```python
from build123d import *

# Parameters (mm, degrees)
SKETCH_1_R               = 30
SKETCH_1_R_2             = 2.75
EXTRUDE_1_DEPTH          = 5
SKETCH_2_R               = 12
EXTRUDE_2_DEPTH          = 10
SKETCH_3_R               = 6
EXTRUDE_3_DEPTH          = 10
SKETCH_5_R               = 5
EXTRUDE_4_DEPTH          = 24.1
SKETCH_6_R               = 2
CUT_EXTRUDE_1_DEPTH      = 10
CUT_EXTRUDE_1_DEPTH_BACK = 10


with BuildPart() as part:
    # Sketch 1 → Extrude 1 (new body)
    with BuildSketch(Plane.XY):
        Circle(SKETCH_1_R)
        with Locations((0, 22.5)):
            Circle(SKETCH_1_R_2, mode=Mode.SUBTRACT)
        with Locations((19.485571585, 11.25)):
            Circle(SKETCH_1_R_2, mode=Mode.SUBTRACT)
        with Locations((19.485571585, -11.25)):
            Circle(SKETCH_1_R_2, mode=Mode.SUBTRACT)
        with Locations((0, -22.5)):
            Circle(SKETCH_1_R_2, mode=Mode.SUBTRACT)
        with Locations((-19.485571585, -11.25)):
            Circle(SKETCH_1_R_2, mode=Mode.SUBTRACT)
        with Locations((-19.485571585, 11.25)):
            Circle(SKETCH_1_R_2, mode=Mode.SUBTRACT)
    extrude(amount=EXTRUDE_1_DEPTH)

    # Sketch 2 → Extrude 2 (add)
    with BuildSketch(Plane.XY.offset(5)):
        Circle(SKETCH_2_R)
    extrude(amount=EXTRUDE_2_DEPTH)

    # Sketch 3 → Extrude 3 (add)
    with BuildSketch(Plane.XY.offset(15)):
        Circle(SKETCH_3_R)
    extrude(amount=EXTRUDE_3_DEPTH)

    # Sketch 5 → Extrude 4 (add)
    with BuildSketch(Plane.XY.offset(25)):
        Circle(SKETCH_5_R)
    extrude(amount=EXTRUDE_4_DEPTH)

    # Sketch 6 → Cut-Extrude 1 (cut, two sides)
    with BuildSketch(Plane(origin=(0, 0, 0), x_dir=(1, 0, 0), z_dir=(0, 1, 0))) as cut_extrude_1_sk:
        with Locations((0, -39.1)):
            Circle(SKETCH_6_R)
    extrude(amount=CUT_EXTRUDE_1_DEPTH, mode=Mode.SUBTRACT)
    extrude(cut_extrude_1_sk.sketch, amount=-CUT_EXTRUDE_1_DEPTH_BACK, mode=Mode.SUBTRACT)


solid = part.part
```
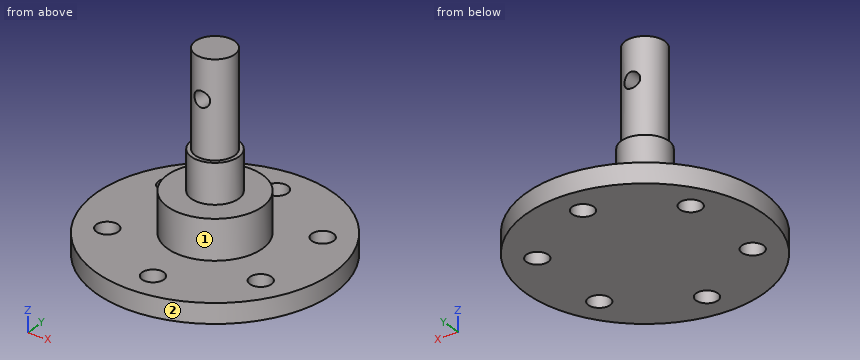
Design review of the part built by this model. Coordinates are the model's own, in mm. Face numbers are marked on the shaded views. A direction names the side the tool comes from. Give positions to 0.01 mm unless a question says otherwise; leave off trailing zeros. Order: outer loops, then holes, each group sorted by start corner. A loop starts at its lowest first (then second) coordinate and runs counter-clockwise, first axis right, second up. Notation, with made-up numbers: (72, -13.75) -> (102, -13.75) arc R31 cw to (102, 24.25) -> close; hole circle Ø2 at (87, 22). An arc over 180 degrees is marked (long way). Write each question's results on one line, items separated by ' | '. Start each with the question number.
Q1. Machinability: for the marked faces 1 and 2, which of the approach directions +Z, -Z, +X, -X, +Y, -Y give a long, thin tool a straight path to every point of the face, cutting with its end or side? Answer none if there is none.
Q2. Add section A-A on x = 0. Give the boundary of the cut face in (y, z), and give its area (3 significant figures).
Q3. Add section D-D on x = -18.5. Give the boundary of the cut face in (y, z).
Q4. Wall thickness on L1, parallel to Y at x = 0, z = 3.05; L2, parallel to X at y = -11, z = 3; L3, parallel to Z at x = 21, y = 16.5: over which ranges is each line inside the solid? List them lowest first. Write a range as from..to.
Q5. For pin 1 (3.5 mm diameter, centred on x = -19.49, y = 11.25, fed in from +Z); pin 2 (2 mm diameter, centred on x = 4, y = 10.5, fed in from +Z); pin 3 (12 mm diameter, centred on x = -5, z = 26.5, fed in from +Y); pin 4 (6 mm diameter, centred on x = -22.5, z = 7.5, fed in from -Y), all flat-tipped, find the tip position at first contact; note any pin that passes through.
Q6. Add section C-C on y = 0. Give the boundary of the cut face in (x, z).
Q7. Add section B-B on y = -13. Give the boundary of the cut face in (x, z).
Found:
1) face 1: +Z | face 2: +Z, -Z
2) outline: (-30, 0) -> (-25.25, 0) -> (-25.25, 5) -> (-30, 5) -> close; (-19.75, 0) -> (19.75, 0) -> (19.75, 5) -> (12, 5) -> (12, 15) -> (6, 15) -> (6, 25) -> (5, 25) -> (5, 37.1) -> (-5, 37.1) -> (-5, 25) -> (-6, 25) -> (-6, 15) -> (-12, 15) -> (-12, 5) -> (-19.75, 5) -> close; (-5, 41.1) -> (5, 41.1) -> (5, 49.1) -> (-5, 49.1) -> close; (25.25, 0) -> (30, 0) -> (30, 5) -> (25.25, 5) -> close | area: 806 mm2
3) outline: (-23.62, 0) -> (-13.82, 0) -> (-13.82, 5) -> (-23.62, 5) -> close; (-8.68, 0) -> (8.68, 0) -> (8.68, 5) -> (-8.68, 5) -> close; (13.82, 0) -> (23.62, 0) -> (23.62, 5) -> (13.82, 5) -> close
4) L1: y = -30..-25.25, -19.75..19.75, 25.25..30 | L2: x = -27.91..-22.22, -16.75..16.75, 22.22..27.91 | L3: z = 0..5
5) pin 1: passes through | pin 2: stops at z = 15 | pin 3: stops at y = 6 | pin 4: stops at y = -21.58
6) outline: (-30, 0) -> (30, 0) -> (30, 5) -> (12, 5) -> (12, 15) -> (6, 15) -> (6, 25) -> (5, 25) -> (5, 49.1) -> (-5, 49.1) -> (-5, 25) -> (-6, 25) -> (-6, 15) -> (-12, 15) -> (-12, 5) -> (-30, 5) -> close; hole circle Ø4 at (0, 39.1)
7) outline: (-27.04, 0) -> (-21.61, 0) -> (-21.61, 5) -> (-27.04, 5) -> close; (-17.36, 0) -> (17.36, 0) -> (17.36, 5) -> (-17.36, 5) -> close; (21.61, 0) -> (27.04, 0) -> (27.04, 5) -> (21.61, 5) -> close
